Autodesk Inventor part; units mm, degrees
ref_plane "YZ Plane" through (0, 0, 0) normal (1, 0, 0) x (0, 1, 0)
ref_plane "XZ Plane" through (0, 0, 0) normal (0, 1, 0) x (-1, 0, 0)
ref_plane "XY Plane" through (0, 0, 0) normal (0, 0, 1) x (1, 0, 0)
sketch "Sketch1" plane through (0, 0, 0) normal (0, 0, 1) x (1, 0, 0)
  line L0 (0, 0) -> (9, 0)
  line L1 (9, 0) -> (9, -1.5)
  line L2 (9, -1.5) -> (7.5, -1.5)
  line L3 (7.5, -1.5) -> (7.5, -31.2)
  line L4 (7.5, -31.2) -> (6, -31.2)
  line L5 (6, -31.2) -> (6, -36.8)
  line L6 (6, -36.8) -> (0, -36.8)
  line L7 (0, -36.8) -> (0, 0)
  dimension "d0" = 9
  dimension "d1" = 1.5
  dimension "d2" = 29.7
  dimension "d3" = 5.6
  dimension "d4" = 7.5
  dimension "d5" = 6
revolve "Revolution1" add sketch "Sketch1" angle 360 about axis through (0, -36.8, 0) along (0, 1, 0)
properties part number "Button"
Geometry check sheet. Reference: the model listing, model coordinates, mm. A direction names the side the tool comes from. Give positions to 0.01 mm unless a question says otherwise; leave off trailing zeros. Write each loop counter-clockwise with the first axis right and the second up, starting at its lowest first coordinate (ties: lowest second). Pieces come first, ordered by that corner, then holes. Notation, with made-up numbers: (-9.75, 35.5) -> (44.25, 35.5) arc R35 ccw to (44.25, 69.5) -> close; hole circle Ø6 at (-34.75, 11.25). An arc over 180 degrees is marked (long way). One line per question, with ' | ' between items.
Item 1: Sectioned sample at B-B, the plane z = 0. Record the boundary of the cut face in (x, y), plus the area to 3 significant figures.
Determined:
outline: (-9, -1.5) -> (-7.5, -1.5) -> (-7.5, -31.2) -> (-6, -31.2) -> (-6, -36.8) -> (6, -36.8) -> (6, -31.2) -> (7.5, -31.2) -> (7.5, -1.5) -> (9, -1.5) -> (9, 0) -> (-9, 0) -> close | area: 540 mm^2
Item 2: Depth check by flat-ended pin: pin 1 (4 mm diameter, centred on x = -2, y = -5, fed in from -Z); pin 2 (5 mm diameter, centred on x = -2.5, y = -28, fed in from +Z); pin 3 (2 mm diameter, centred on y = -22.5, z = -5, fed in from -X). Enter the tip coordinate at first touch or a pass-through.
Determined:
pin 1: z = -7.5 | pin 2: z = 7.5 | pin 3: x = -6.34
Item 3: Sectioned sample at A-A, the plane x = 0. Record the boundary of the cut face in (y, z), plus the area to 3 significant figures.
Determined:
outline: (-36.8, -6) -> (-31.2, -6) -> (-31.2, -7.5) -> (-1.5, -7.5) -> (-1.5, -9) -> (0, -9) -> (0, 9) -> (-1.5, 9) -> (-1.5, 7.5) -> (-31.2, 7.5) -> (-31.2, 6) -> (-36.8, 6) -> close | area: 540 mm^2
Item 4: Scan lines: line 1 along X through (y, z) = (-31, 0); line 2 along X through (y, z) = (-21.5, 3.25); line 3 along Y through (x, z) = (3.75, -5). Record each from-to range of solid material in increasing order.
Determined:
line 1: -7.5 to 7.5 | line 2: -6.76 to 6.76 | line 3: -31.2 to 0
Item 5: Sectioned sample at D-D, the plane x = -6.75. Record the boundary of the cut face in (y, z), plus the area to 3 significant figures.
Determined:
outline: (-31.2, -3.27) -> (-1.5, -3.27) -> (-1.5, -5.95) -> (0, -5.95) -> (0, 5.95) -> (-1.5, 5.95) -> (-1.5, 3.27) -> (-31.2, 3.27) -> close | area: 212 mm^2
Item 6: Access from +Z, -Z, +X, -X, +Y, -Y to the whole of each face (thin tool, end or side, straight path). Record for faces 1 (the cylindrical face through (-1.172, -0.76, 8.923)), 2 (the flat face through (-2, -1.5, -7.4)).
Determined:
face 1: +Y, -Y | face 2: -Y
Item 7: Sectioned sample at C-C, the plane y = -9.5. Record the boundary of the cut face in (x, z), plus the area to 3 significant figures.
Determined:
outline: circle Ø15 at (0, 0) | area: 177 mm^2
